```python
from build123d import *

# Parameters (mm, degrees)
REVOLVE_2_ANGLE     = 14
SKETCH_5_W          = 44.686573774
SKETCH_5_H          = 93.829393492
CUT_EXTRUDE_1_DEPTH = 50
SKETCH_6_W          = 25.08892812
SKETCH_6_H          = 77.533839386
CUT_EXTRUDE_2_DEPTH = 39


with BuildPart() as part:
    # 草图3 → 旋转2 (revolve)
    with BuildSketch(Plane(origin=(0, 0, 0), x_dir=(1, 0, 0), z_dir=(0, 1, 0))):
        with BuildLine():
            Line((-30, 0), (30, 0))
            ThreePointArc((30, 0), (0, 30), (-30, 0))
        make_face()
    revolve(axis=Axis((-30, 0, 0), (1, 0, 0)), revolution_arc=REVOLVE_2_ANGLE)

    # 草图5 → 切除-拉伸1 (cut)
    with BuildSketch(Plane(origin=(0, 0, 0), x_dir=(0, 1, 0), z_dir=(-0.8660254037844416, 0, -0.49999999999999495))):
        Rectangle(SKETCH_5_W, SKETCH_5_H)
    extrude(amount=-CUT_EXTRUDE_1_DEPTH, mode=Mode.SUBTRACT)

    # 草图6 → 切除-拉伸2 (cut)
    with BuildSketch(Plane(origin=(0, 0, 0), x_dir=(0, 1, 0), z_dir=(-0.8660254037844416, 0, 0.49999999999999495))):
        Rectangle(SKETCH_6_W, SKETCH_6_H)
    extrude(amount=CUT_EXTRUDE_2_DEPTH, mode=Mode.SUBTRACT)


solid = part.part
```
Geometry check sheet. Reference: the model listing, model coordinates, mm. Give positions to 0.01 mm unless a question says otherwise; leave off trailing zeros. Write each loop counter-clockwise with the first axis right and the second up, starting at its lowest first coordinate (ties: lowest second). Pieces come first, ordered by that corner, then holes.
1) Gauge pin test, flat ends, axial feed: pin 1 (1.5 mm diameter, centred on x = -3, z = -3, fed in from +Y); pin 2 (3 mm diameter, centred on x = 7, y = 5.5, fed in from -Z); pin 3 (2 mm diameter, centred on x = -6, y = 1.5, fed in from -Z); pin 4 (2 mm diameter, centred on y = 4.5, z = -17.5, fed in from -X). Record the tip position at first contact, or that the pin passes through.
2) Section check A-A, the plane z = -14.75. Record the boundary of the cut face in (x, y).
3) Section check B-B, the plane x = -2. Record the boundary of the cut face in (y, z).
4) Material ranges on L1, parallel to Z at x = -6.25, y = 1.5; L2, parallel to Y at x = -3.5, z = -12.5; L3, parallel to Y at x = 2.5, z = -15, recorded low to high.
Computed:
1. pin 1: passes through
1. pin 2: stops at z = -29.07
1. pin 3: stops at z = -29.55
1. pin 4: stops at x = -10.68
2. outline: (-8.52, 0) - (8.52, 0) - (8.52, 3.68) - (-8.52, 3.68) - close
3. outline: (0, -29.93) arc R29.93 ccw to (7.24, -29.04) - (0.86, -3.46) - (0, -3.46) - close
4. L1: z = -29.3 to -10.83
4. L2: y = 0 to 3.12
4. L3: y = 0 to 3.74
